Input: dimensioned drawing with shaded views. Units: mm. Origin: part minimum x, y, z. Coordinates: 2 decimals unless noted, no trailing zeros. Put each result on its own line as item: value. Start each with the question number.
1) Contact query for flat-ended pins moving along their axis: pin 1 Ø5.5 at (x, y) = (265.9, 104.78) entering from -Z; pin 2 Ø3 at (x, z) = (174.5, 3.5) entering from +Y; pin 3 Ø3 at (x, z) = (249.5, 3) entering from +Y (3 decimals); pin 4 Ø1 at (x, z) = (242.5, 4.5) entering from -Y (3 decimals). Output: stop coordinate, or through.
2) Section A-A on x = 12.7. Count the separate pieces of the cut face and the enclosed holes in it, and give its area (3 significant figures).
3) Material intervals for line 1 along X through (y, z) = (77, 5.25) (1 decimal); line 2 along Y through (x, z) = (22, 1) (1 decimal); line 3 along X through (y, z) = (92, 1.25) (1 decimal), sorted ascending. Write a range as from..to.
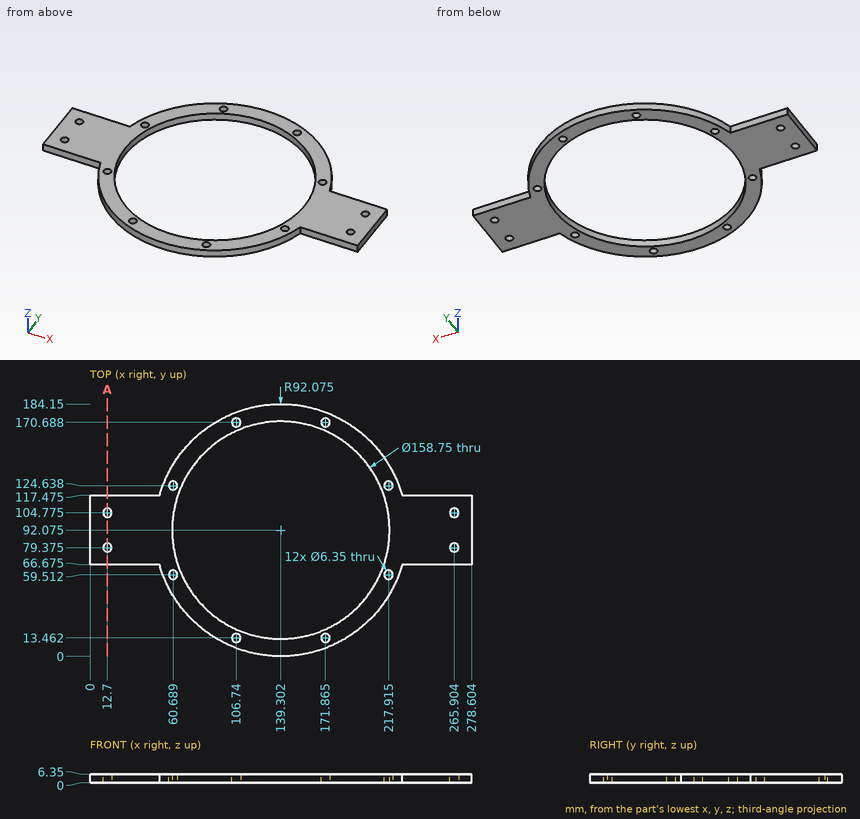
Answer block:
1. pin 1: passes through
1. pin 2: stops at y = 177.76
1. pin 3: stops at y = 117.475
1. pin 4: stops at y = 66.675
2. separate pieces: 3
2. enclosed holes: 0
2. area: 242 mm²
3. line 1: x = 0..10.6, 14.8..61.4, 217.2..263.8, 268..278.6
3. line 2: y = 66.7..117.5
3. line 3: x = 0..59.9, 218.7..278.6
